Could you check a few things on this model? Use its own coordinates, in mm. Give positions to 0.01 mm unless a question says otherwise; leave off trailing zeros. Loops run counter-clockwise (first coordinate to the right, second up) from the corner with the lowest first, then second, coordinate; pieces in that order, holes last.
1. Imagine slicing it at A-A (y = -45.5). List the corners of the cut face in (x, z) for me, plus the area to 3 significant figures.
2. Imagine slicing it at C-C (z = 0.3). Count the separate pieces of the cut face and the enclosed holes in it, plus the area to 3 significant figures.
3. Thinking about a two-plate mould opening in Y: for faces 1 (the flat face through (-2, -15, 2)), 2 (the cylindrical face through (34.43, 1.51, 0.99)), which applies, +Y half, -Y half, draft (parallel to the pull), parting line (faces both ways), or undercut?
4. I need wall thicknesses on line 1 along X through (y, z) = (8, 1.75); line 2 along Y through (x, z) = (48.5, 0.3); line 3 along Y through (x, z) = (-39.5, 0.5). Which ranges of each line are inside material? Lowest first, please.
5. Imagine slicing it at B-B (x = -37). List the corners of the cut face in (y, z) for me, plus the area to 3 significant figures.
```python
from build123d import *

# Parameters (mm, degrees)
F0_W     = 41
F0_H     = 106
F0_R     = 6
F0_R_2   = 2
F0_R_3   = 9.5
F0_W_2   = 0.927996
F1_DEPTH = 2


with BuildPart() as f1:
    # F0 (on Top) → F1 (new body)
    with BuildSketch(Plane.XY):
        with Locations((-42.758821, -4.311392)):
            Rectangle(F0_W, F0_H)
        with Locations((-48.35481, -36.657964)):
            Circle(F0_R, mode=Mode.SUBTRACT)
        with BuildLine():
            ThreePointArc((-40.758821, -31.657964), (-46.365975, -28.882496), (-49.258821, -23.334988))
            Line((-49.258821, -23.334988), (-30.258821, -23.692439))
            Line((-30.258821, -23.692439), (-30.258821, -49.692439))
            Line((-30.258821, -49.692439), (-49.258821, -49.98094))
            ThreePointArc((-49.258821, -49.98094), (-46.365975, -44.433432), (-40.758821, -41.657964))
            Line((-40.758821, -41.657964), (-40.758821, -31.657964))
        make_face(mode=Mode.SUBTRACT)
        with Locations((-53.414003, -21.625079)):
            Circle(F0_R_2, mode=Mode.SUBTRACT)
        with Locations((-53.414003, -3.311392)):
            Circle(F0_R_2, mode=Mode.SUBTRACT)
        with Locations((-40.008821, 1.088608)):
            Circle(F0_R_3, mode=Mode.SUBTRACT)
        with Locations((-53.414003, 15.002295)):
            Circle(F0_R_2, mode=Mode.SUBTRACT)
        with Locations((-48.35481, 30.03518)):
            Circle(F0_R, mode=Mode.SUBTRACT)
        with BuildLine():
            ThreePointArc((-40.758821, 35.03518), (-46.365975, 37.810648), (-49.258821, 43.358156))
            Line((-49.258821, 43.358156), (-30.258821, 43.069655))
            Line((-30.258821, 43.069655), (-30.258821, 27.304233))
            Line((-30.258821, 27.304233), (-28.396592, 22.957894))
            ThreePointArc((-28.396592, 22.957894), (-27.630572, 21.936268), (-27.358821, 20.688608))
            ThreePointArc((-27.358821, 20.688608), (-28.202435, 18.602943), (-30.258821, 17.690275))
            Line((-30.258821, 17.690275), (-30.258821, 17.069655))
            Line((-30.258821, 17.069655), (-49.258821, 16.712204))
            ThreePointArc((-49.258821, 16.712204), (-46.365975, 22.259712), (-40.758821, 25.03518))
            Line((-40.758821, 25.03518), (-40.758821, 35.03518))
        make_face(mode=Mode.SUBTRACT)
        with Locations((-21.794823, -4.311392)):
            Rectangle(F0_W_2, F0_H)
        with Locations((-0.830825, -4.311392)):
            Rectangle(F0_W, F0_H)
        with Locations((-6.426815, -36.657964)):
            Circle(F0_R, mode=Mode.SUBTRACT)
        with Locations((-11.486007, -21.625079)):
            Circle(F0_R_2, mode=Mode.SUBTRACT)
        with BuildLine():
            ThreePointArc((1.169175, -31.657964), (-4.437979, -28.882496), (-7.330825, -23.334988))
            Line((-7.330825, -23.334988), (11.669175, -23.692439))
            Line((11.669175, -23.692439), (11.669175, -49.692439))
            Line((11.669175, -49.692439), (-7.330825, -49.98094))
            ThreePointArc((-7.330825, -49.98094), (-4.437979, -44.433432), (1.169175, -41.657964))
            Line((1.169175, -41.657964), (1.169175, -31.657964))
        make_face(mode=Mode.SUBTRACT)
        with Locations((-11.486007, -3.311392)):
            Circle(F0_R_2, mode=Mode.SUBTRACT)
        with Locations((-11.486007, 15.002295)):
            Circle(F0_R_2, mode=Mode.SUBTRACT)
        with Locations((-6.426815, 30.03518)):
            Circle(F0_R, mode=Mode.SUBTRACT)
        with Locations((1.919175, 1.088608)):
            Circle(F0_R_3, mode=Mode.SUBTRACT)
        with BuildLine():
            ThreePointArc((1.169175, 35.03518), (-4.437979, 37.810648), (-7.330825, 43.358156))
            Line((-7.330825, 43.358156), (11.669175, 43.069655))
            Line((11.669175, 43.069655), (11.669175, 27.304233))
            Line((11.669175, 27.304233), (13.531403, 22.957894))
            ThreePointArc((13.531403, 22.957894), (14.297424, 21.936268), (14.569175, 20.688608))
            ThreePointArc((14.569175, 20.688608), (13.725561, 18.602943), (11.669175, 17.690275))
            Line((11.669175, 17.690275), (11.669175, 17.069655))
            Line((11.669175, 17.069655), (-7.330825, 16.712204))
            ThreePointArc((-7.330825, 16.712204), (-4.437979, 22.259712), (1.169175, 25.03518))
            Line((1.169175, 25.03518), (1.169175, 35.03518))
        make_face(mode=Mode.SUBTRACT)
        Polygon((20.669173, 48.688607), (19.669175, 48.688608), (19.669175, -57.311392), (20.669173, -57.311393), align=None)
        with Locations((41.169173, -4.311393)):
            Rectangle(F0_W, F0_H)
        with Locations((35.573184, -36.657965)):
            Circle(F0_R, mode=Mode.SUBTRACT)
        with BuildLine():
            ThreePointArc((43.169173, -31.657965), (37.562019, -28.882497), (34.669173, -23.33499))
            Line((34.669173, -23.33499), (53.669173, -23.692441))
            Line((53.669173, -23.692441), (53.669173, -49.692441))
            Line((53.669173, -49.692441), (34.669173, -49.980941))
            ThreePointArc((34.669173, -49.980941), (37.562019, -44.433434), (43.169173, -41.657965))
            Line((43.169173, -41.657965), (43.169173, -31.657965))
        make_face(mode=Mode.SUBTRACT)
        with Locations((30.513992, -21.62508)):
            Circle(F0_R_2, mode=Mode.SUBTRACT)
        with Locations((30.513992, -3.311393)):
            Circle(F0_R_2, mode=Mode.SUBTRACT)
        with Locations((43.919173, 1.088607)):
            Circle(F0_R_3, mode=Mode.SUBTRACT)
        with Locations((30.513992, 15.002294)):
            Circle(F0_R_2, mode=Mode.SUBTRACT)
        with Locations((35.573184, 30.035179)):
            Circle(F0_R, mode=Mode.SUBTRACT)
        with BuildLine():
            ThreePointArc((43.169173, 35.035179), (37.562019, 37.810647), (34.669173, 43.358155))
            Line((34.669173, 43.358155), (53.669173, 43.069654))
            Line((53.669173, 43.069654), (53.669173, 27.304232))
            Line((53.669173, 27.304232), (55.531402, 22.957893))
            ThreePointArc((55.531402, 22.957893), (56.297423, 21.936267), (56.569173, 20.688607))
            ThreePointArc((56.569173, 20.688607), (55.725559, 18.602941), (53.669173, 17.690274))
            Line((53.669173, 17.690274), (53.669173, 17.069654))
            Line((53.669173, 17.069654), (34.669173, 16.712203))
            ThreePointArc((34.669173, 16.712203), (37.562019, 22.259711), (43.169173, 25.035179))
            Line((43.169173, 25.035179), (43.169173, 35.035179))
        make_face(mode=Mode.SUBTRACT)
    extrude(amount=F1_DEPTH)


solid = f1.part
```
Derived:
1. outline: (-63.26, 0) - (-47.31, 0) - (-47.31, 2) - (-63.26, 2) - close; (-30.26, 0) - (-5.38, 0) - (-5.38, 2) - (-30.26, 2) - close; (11.67, 0) - (36.62, 0) - (36.62, 2) - (11.67, 2) - close; (53.67, 0) - (61.67, 0) - (61.67, 2) - (53.67, 2) - close
1. area: 148 mm2
2. separate pieces: 1
2. enclosed holes: 24
2. area: 9,300 mm2
3. face 1: draft
3. face 2: undercut
4. line 1: x = -63.26 to -46.53, -33.49 to -4.6, 8.44 to 37.4, 50.44 to 61.67
4. line 2: y = -57.31 to -49.77, -23.6 to -7.23, 9.41 to 16.97, 43.15 to 48.69
4. line 3: y = -57.31 to -49.83, -23.52 to -8.4, 10.57 to 16.9, 43.21 to 48.69
5. outline: (-57.31, 0) - (-49.79, 0) - (-49.79, 2) - (-57.31, 2) - close; (-23.57, 0) - (-7.92, 0) - (-7.92, 2) - (-23.57, 2) - close; (10.1, 0) - (16.94, 0) - (16.94, 2) - (10.1, 2) - close; (43.17, 0) - (48.69, 0) - (48.69, 2) - (43.17, 2) - close
5. area: 71.0 mm2
